Can you work these out from the drawing? Everything is in mm from the part's minimum corner. A direction names the side the tool comes from. Give positions to 0.01 mm unless a question says otherwise; leave off trailing zeros. Write each loop counter-clockwise with the first axis right and the second up, starting at its lowest first coordinate (ties: lowest second). Pieces come first, ordered by that corner, then holes. Notation, with made-up numbers: (-20, 64.5) - (10, 64.5) arc R19 ccw to (10, 85.5) - close; hole circle Ø9 at (88, 36.25). An arc over 180 degrees is marked (long way). Use a Markdown table: item, result.
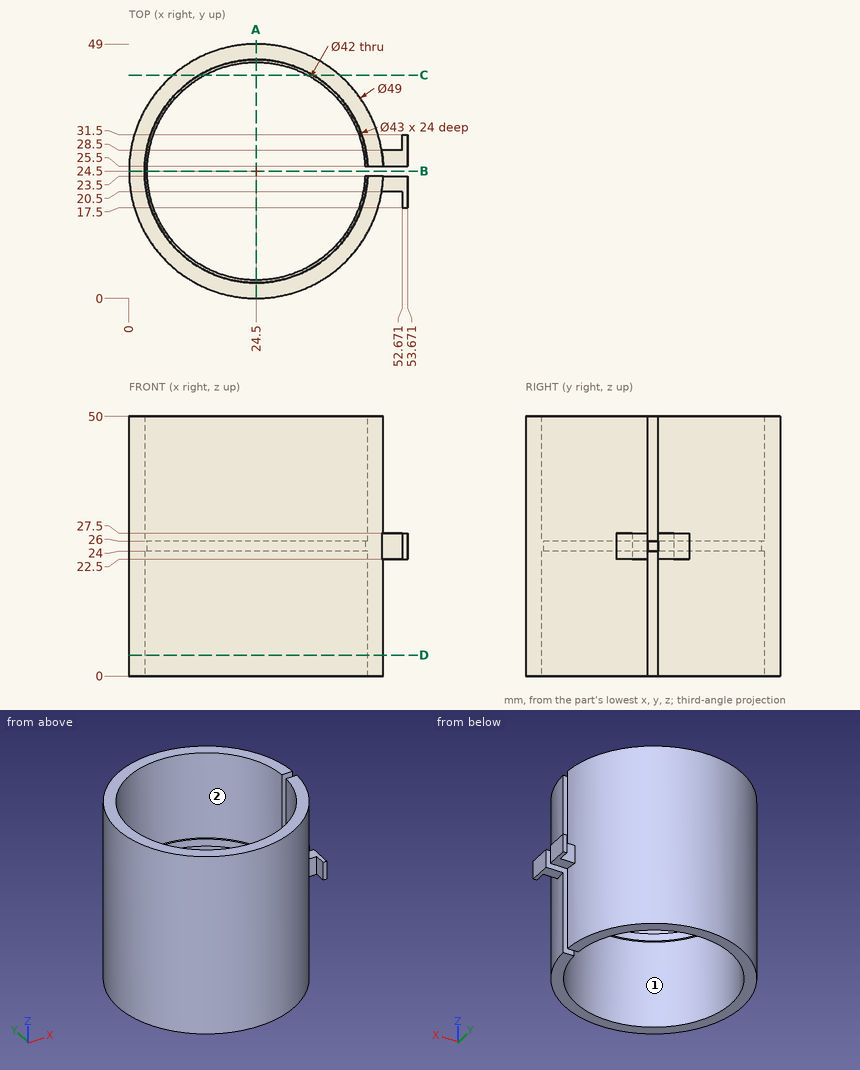
Item 1: Will these pins go through, and if not, where does the flat tip stop? pin 1 Ø2.5 at (x, y) = (51.5, 27.5) entering from +Z; pin 2 Ø2.5 at (x, y) = (52.5, 21) entering from -Z; pin 3 Ø3.5 at (y, z) = (30.5, 26) entering from -X.
Values:
| item | result |
|---|---|
| pin 1 | stops at z = 27.5 |
| pin 2 | stops at z = 22.5 |
| pin 3 | stops at x = 0.37 |
Item 2: If we section it at A-A, the plane x = 24.5: Write out the boundary of the cut face in (y, z).
Values:
| item | result |
|---|---|
| outline | (0, 0) - (3, 0) - (3, 24) - (3.5, 24) - (3.5, 26) - (3, 26) - (3, 50) - (0, 50) - close; (45.5, 24) - (46, 24) - (46, 0) - (49, 0) - (49, 50) - (46, 50) - (46, 26) - (45.5, 26) - close |
Item 3: If we section it at D-D, the plane z = 4: Write out the boundary of the cut face in (x, y).
Values:
| item | result |
|---|---|
| outline | (45.98, 23.5) arc R21.5 cw (long way) to (45.98, 25.5) - (48.98, 25.5) arc R24.5 ccw (long way) to (48.98, 23.5) - close |
Item 4: I need wall thicknesses on line 1 along Y through (x, z) = (24.5, 44.25); line 2 along Y through (x, z) = (24.5, 25.6); line 3 along X through (y, z) = (24.5, 5.75). Which ranges of each line are inside material? Lowest first, please. Write a range as [from, to].
Values:
| item | result |
|---|---|
| line 1 | y = [0, 3], [46, 49] |
| line 2 | y = [0, 3.5], [45.5, 49] |
| line 3 | x = [0, 3] |
Item 5: For the marked faces 1 and 2, which set-ups out of +Z, -Z, +X, -X, +Y, -Y let a thin tool reach every point of the face, with its end or its side?
Values:
| item | result |
|---|---|
| face 1 | -Z |
| face 2 | +Z |
Item 6: If we section it at C-C, the plane y = 43: Write out the boundary of the cut face in (x, z).
Values:
| item | result |
|---|---|
| outline | (8.44, 0) - (13.55, 0) - (13.55, 24) - (14.56, 24) - (14.56, 26) - (13.55, 26) - (13.55, 50) - (8.44, 50) - close; (34.44, 24) - (35.45, 24) - (35.45, 0) - (40.56, 0) - (40.56, 50) - (35.45, 50) - (35.45, 26) - (34.44, 26) - close |
Item 7: If we section it at B-B, the plane y = 24.5: Write out the boundary of the cut face in (x, z).
Values:
| item | result |
|---|---|
| outline | (0, 0) - (3, 0) - (3, 24) - (3.5, 24) - (3.5, 26) - (3, 26) - (3, 50) - (0, 50) - close |
